Autodesk Inventor part; units mm, degrees
ref_plane "YZ Plane" through (0, 0, 0) normal (1, 0, 0) x (0, 1, 0)
ref_plane "XZ Plane" through (0, 0, 0) normal (0, 1, 0) x (-1, 0, 0)
ref_plane "XY Plane" through (0, 0, 0) normal (0, 0, 1) x (1, 0, 0)
sketch "Sketch1" plane through (0, 0, 0) normal (0, 1, 0) x (-1, 0, 0)
  line L0 (-25, 50) -> (25, 50)
  line L1 (25, 50) -> (25, -50)
  line L2 (25, -50) -> (-25, -50)
  line L3 (-25, -50) -> (-25, 50)
  line L4 (-25, 50) -> (25, -50) construction
  line L5 (25, 50) -> (-25, -50) construction
  line L6 (-25, 50) -> (-25, 40)
  line L7 (-25, 40) -> (-15, 40)
  circle A0 centre (-15, 40) radius 4
  line L8 (-25, -50) -> (-25, -40)
  line L9 (-25, -40) -> (-15, -40)
  circle A1 centre (-15, -40) radius 4
  point P0 (0, 0)
  dimension "d0" = 50
  dimension "d1" = 100
  dimension "d8" = 10
  dimension "d9" = 10
  dimension "d10" = 8
  dimension "d11" = 10
  dimension "d12" = 10
  dimension "d13" = 8
extrude "Extrusion2" add sketch "Sketch1" along normal blind 2
properties part number "H"
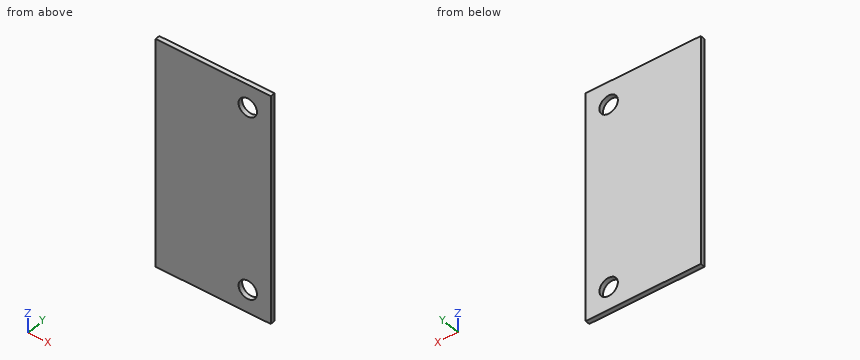
Geometry check sheet. Reference: the model listing, model coordinates, mm. Round coordinates to 2 decimals unless told otherwise and drop trailing zeros. Loops run counter-clockwise (first coordinate to the right, second up) from the corner with the lowest first, then second, coordinate; pieces in that order, holes last.
Item 1: Cross-section at B-B on x = 15. Record the boundary of the cut face in (y, z), then the cut area to 3 significant figures.
Item 2: Cross-section at D-D on z = 39. Record the boundary of the cut face in (x, y).
Item 3: Cross-section at C-C on y = 1.25. Record the boundary of the cut face in (x, z).
Item 4: Gauge pin test, flat end, axial feed: pin 1 (5 mm diameter, centred on x = 15, z = 40, fed in from +Y). Record the tip position at first contact, or that the pin passes through.
Item 5: Cross-section at A-A on z = -40. Record the boundary of the cut face in (x, y), then the cut area to 3 significant figures.
Item 6: Thickness scan on line 1 (Z direction, x = 15, y = 1); line 2 (X direction, y = 0.1, z = 40.5). Record the ranges inside material, lowest first.
Answer sheet:
1. outline: (0, -50) - (2, -50) - (2, -44) - (0, -44) - close; (0, -36) - (2, -36) - (2, 36) - (0, 36) - close; (0, 44) - (2, 44) - (2, 50) - (0, 50) - close
1. area: 168 mm2
2. outline: (-25, 0) - (11.13, 0) - (11.13, 2) - (-25, 2) - close; (18.87, 0) - (25, 0) - (25, 2) - (18.87, 2) - close
3. outline: (-25, -50) - (25, -50) - (25, 50) - (-25, 50) - close; hole circle Ø8 at (15, -40); hole circle Ø8 at (15, 40)
4. pin 1: passes through
5. outline: (-25, 0) - (11, 0) - (11, 2) - (-25, 2) - close; (19, 0) - (25, 0) - (25, 2) - (19, 2) - close
5. area: 84.0 mm2
6. line 1: z = -50 to -44, -36 to 36, 44 to 50
6. line 2: x = -25 to 11.03, 18.97 to 25
